from build123d import *

# Parameters (mm, degrees)
F3_DEPTH = 38.1
F4_R     = 6.35
F5_DEPTH = 38.101


with BuildPart() as f3:
    # F2 (on Front) → F3 (new body)
    with BuildSketch(Plane.XZ):
        with BuildLine():
            Line((209.46872, 55.997023), (0, 55.997023))
            ThreePointArc((0, 55.997023), (-55.997023, 0), (0, -55.997023))
            Line((0, -55.997023), (209.46872, -55.997023))
            ThreePointArc((209.46872, -55.997023), (265.465743, 0), (209.46872, 55.997023))
        make_face()
        with BuildLine():
            ThreePointArc((-6.55809, 47.171306), (-3.286882, 47.511441), (0, 47.625))
            Line((0, 47.625), (6.591117, 47.625))
            ThreePointArc((6.591117, 47.625), (14.96314, 39.252977), (23.335163, 47.625))
            Line((23.335163, 47.625), (36.514857, 47.625))
            ThreePointArc((36.514857, 47.625), (44.88688, 39.252977), (53.258903, 47.625))
            Line((53.258903, 47.625), (66.438597, 47.625))
            ThreePointArc((66.438597, 47.625), (74.81062, 39.252977), (83.182643, 47.625))
            Line((83.182643, 47.625), (96.362337, 47.625))
            ThreePointArc((96.362337, 47.625), (104.73436, 39.252977), (113.106383, 47.625))
            Line((113.106383, 47.625), (126.286077, 47.625))
            ThreePointArc((126.286077, 47.625), (134.6581, 39.252977), (143.030123, 47.625))
            Line((143.030123, 47.625), (156.209817, 47.625))
            ThreePointArc((156.209817, 47.625), (164.58184, 39.252977), (172.953863, 47.625))
            Line((172.953863, 47.625), (186.133557, 47.625))
            ThreePointArc((186.133557, 47.625), (194.50558, 39.252977), (202.877603, 47.625))
            Line((202.877603, 47.625), (209.46872, 47.625))
            ThreePointArc((209.46872, 47.625), (212.755602, 47.511441), (216.02681, 47.171306))
            ThreePointArc((216.02681, 47.171306), (221.598557, 37.3318), (231.889711, 42.017137))
            ThreePointArc((231.889711, 42.017137), (237.461993, 38.529434), (242.500924, 34.307639))
            ThreePointArc((242.500924, 34.307639), (241.225046, 23.072321), (252.304736, 20.813849))
            ThreePointArc((252.304736, 20.813849), (254.762787, 14.716934), (256.357859, 8.339621))
            ThreePointArc((256.357859, 8.339621), (248.721697, 0), (256.357859, -8.339621))
            ThreePointArc((256.357859, -8.339621), (254.762787, -14.716934), (252.304736, -20.813849))
            ThreePointArc((252.304736, -20.813849), (241.225046, -23.072321), (242.500924, -34.307639))
            ThreePointArc((242.500924, -34.307639), (237.461993, -38.529434), (231.889711, -42.017137))
            ThreePointArc((231.889711, -42.017137), (221.598557, -37.3318), (216.02681, -47.171306))
            ThreePointArc((216.02681, -47.171306), (212.755602, -47.511441), (209.46872, -47.625))
            Line((209.46872, -47.625), (202.877603, -47.625))
            ThreePointArc((202.877603, -47.625), (194.50558, -39.252977), (186.133557, -47.625))
            Line((186.133557, -47.625), (172.953863, -47.625))
            ThreePointArc((172.953863, -47.625), (164.58184, -39.252977), (156.209817, -47.625))
            Line((156.209817, -47.625), (143.030123, -47.625))
            ThreePointArc((143.030123, -47.625), (134.6581, -39.252977), (126.286077, -47.625))
            Line((126.286077, -47.625), (113.106383, -47.625))
            ThreePointArc((113.106383, -47.625), (104.73436, -39.252977), (96.362337, -47.625))
            Line((96.362337, -47.625), (83.182643, -47.625))
            ThreePointArc((83.182643, -47.625), (74.81062, -39.252977), (66.438597, -47.625))
            Line((66.438597, -47.625), (53.258903, -47.625))
            ThreePointArc((53.258903, -47.625), (44.88688, -39.252977), (36.514857, -47.625))
            Line((36.514857, -47.625), (23.335163, -47.625))
            ThreePointArc((23.335163, -47.625), (14.96314, -39.252977), (6.591117, -47.625))
            Line((6.591117, -47.625), (0, -47.625))
            ThreePointArc((0, -47.625), (-3.286882, -47.511441), (-6.55809, -47.171306))
            ThreePointArc((-6.55809, -47.171306), (-12.129837, -37.3318), (-22.420991, -42.017137))
            ThreePointArc((-22.420991, -42.017137), (-27.993273, -38.529434), (-33.032204, -34.307639))
            ThreePointArc((-33.032204, -34.307639), (-31.756326, -23.072321), (-42.836016, -20.813849))
            ThreePointArc((-42.836016, -20.813849), (-45.294067, -14.716934), (-46.889139, -8.339621))
            ThreePointArc((-46.889139, -8.339621), (-39.252977, 0), (-46.889139, 8.339621))
            ThreePointArc((-46.889139, 8.339621), (-45.294067, 14.716934), (-42.836016, 20.813849))
            ThreePointArc((-42.836016, 20.813849), (-31.756326, 23.072321), (-33.032204, 34.307639))
            ThreePointArc((-33.032204, 34.307639), (-27.993273, 38.529434), (-22.420991, 42.017137))
            ThreePointArc((-22.420991, 42.017137), (-12.129837, 37.3318), (-6.55809, 47.171306))
        make_face(mode=Mode.SUBTRACT)
    extrude(amount=-F3_DEPTH)

    # F4 (on face) → F5 (cut, through all)
    with BuildSketch(Plane.XZ):
        with Locations((-17.304032, 53.256333)):
            Circle(F4_R)
        with Locations((14.96314, 55.997023)):
            Circle(F4_R)
        with Locations((44.88688, 55.997023)):
            Circle(F4_R)
        with Locations((74.81062, 55.997023)):
            Circle(F4_R)
        with Locations((104.73436, 55.997023)):
            Circle(F4_R)
        with Locations((-45.302543, 32.914224)):
            Circle(F4_R)
        with Locations((-55.997023, 0)):
            Circle(F4_R)
        with Locations((265.465743, 0)):
            Circle(F4_R)
        with Locations((254.771263, 32.914224)):
            Circle(F4_R)
        with Locations((226.772752, 53.256333)):
            Circle(F4_R)
        with Locations((194.50558, 55.997023)):
            Circle(F4_R)
        with Locations((164.58184, 55.997023)):
            Circle(F4_R)
        with Locations((134.6581, 55.997023)):
            Circle(F4_R)
        with Locations((-45.302543, -32.914224)):
            Circle(F4_R)
        with Locations((-17.304032, -53.256333)):
            Circle(F4_R)
        with Locations((14.96314, -55.997023)):
            Circle(F4_R)
        with Locations((44.88688, -55.997023)):
            Circle(F4_R)
        with Locations((74.81062, -55.997023)):
            Circle(F4_R)
        with Locations((104.73436, -55.997023)):
            Circle(F4_R)
        with Locations((134.6581, -55.997023)):
            Circle(F4_R)
        with Locations((164.58184, -55.997023)):
            Circle(F4_R)
        with Locations((194.50558, -55.997023)):
            Circle(F4_R)
        with Locations((226.772752, -53.256333)):
            Circle(F4_R)
        with Locations((254.771263, -32.914224)):
            Circle(F4_R)
    extrude(amount=-F5_DEPTH, mode=Mode.SUBTRACT)


solid = f3.part
The listing builds one solid part. Answer for the finished solid, in the listing's coordinates (mm). A direction names the side the tool comes from. Give positions to 0.01 mm unless a question says otherwise; leave off trailing zeros. Order: outer loops, then holes, each group sorted by start corner. A loop starts at its lowest first (then second) coordinate and runs counter-clockwise, first axis right, second up. Notation, with made-up numbers: (-27.75, -26) - (-19.75, -26) arc R19 cw to (-19.75, -20) - close; hole circle Ø6 at (-37.75, 88). An arc over 180 degrees is marked (long way). One line per item, written item: value. Start each with the question number.
1) Find the intervals of material crossed by L1, parallel to Z at x = 24.5, y = 8 (3 decimals); L2, parallel to Z at x = 104.5, y = 25.5; L3, parallel to X at y = 31.5, z = 20.5, in increasing order.
2) Given pin 1 Ø1 at (x, y) = (14, 7.5) entering from +Z; pin 2 Ø2 at (y, z) = (6, -12) entering from -X; pin 3 Ø1 at (x, y) = (48.5, 12.5) entering from -Z; pin 4 Ø12 at (x, z) = (131, -28.5) entering from -Y (3 decimals), each flat-ended and moving along its own axis, determine where each tip first touches the part or whether it passes through.
3) A cutting plane is placed at A-A on z = 0. Give the vertices of the cut face in (x, y).
4) A cutting plane is placed at B-B on z = 16. Give the vertices of the cut face in (x, y).
5) A tool of negligible diameter and unlimited length cuts with its end or side. For faces 4 (the face through (104.918, 18.783, -39.255)), 5 (the face through (194.37, 18.78, 49.65)), from which of +Z, -Z, +X, -X, +Y, -Y can it reach the whole face along a straight path? Write none if from no direction.
6) The mould has two halves that part along X. Classify faces 1 (the face through (120, 19, -55.997)), 2 (the face through (-28.068, 18.783, 38.475)), 3 (the face through (-5.532, 18.783, 55.723)): released by +X, released by -X, zero draft, split by the parting line, or undercut.
Answer sheet:
1. L1: z = -55.997 to -47.625, 47.625 to 55.997
1. L2: z = -49.65 to -39.26, 39.26 to 49.65
1. L3: x = -52.11 to -42.99, -42.26 to -34.8, 244.26 to 251.73, 252.46 to 261.58
2. pin 1: stops at z = 49.82
2. pin 2: stops at x = -54.91
2. pin 3: stops at z = -51.16
2. pin 4: passes through
3. outline: (-49.65, 0) - (-39.25, 0) - (-39.25, 38.1) - (-49.65, 38.1) - close; (248.72, 0) - (259.12, 0) - (259.12, 38.1) - (248.72, 38.1) - close
4. outline: (-53.66, 0) - (-44.86, 0) - (-44.86, 38.1) - (-53.66, 38.1) - close; (254.33, 0) - (263.13, 0) - (263.13, 38.1) - (254.33, 38.1) - close
5. face 4: +Y, -Y
5. face 5: +Z, +Y, -Y
6. face 1: zero draft
6. face 2: undercut
6. face 3: released by -X
